For this review, take the finished solid that the model builds, in its own axes (mm). A direction names the side the tool comes from. Coordinates: 2 decimals unless noted, no trailing zeros. Write each loop counter-clockwise with the first axis right and the second up, starting at its lowest first coordinate (ties: lowest second). Pieces come first, ordered by that corner, then holes. Notation, with made-up numbers: M -13,40.5 L 44,40.5 A13 cw 44,47.5 Z; hole C -30.75,22 d10. An arc over 180 degrees is marked long. One line per question, with ' | ' between items.
from build123d import *

# Parameters (mm, degrees)
BOSS_EXTRUDE1_DEPTH  = 20
SKETCH2_W            = 20
SKETCH2_H            = 22
BOSS_EXTRUDE2_DEPTH  = 2.2
BOSS_EXTRUDE3_DEPTH  = 2
SKETCH5_R            = 2.5
BOSS_EXTRUDE4_DEPTH  = 4
FILLET1_R            = 1
FILLET2_R            = 1
FILLET1_OF_MIRROR1_R = 1
FILLET2_OF_MIRROR1_R = 1
SKETCH6_R            = 2
CUT_EXTRUDE1_DEPTH   = 38.406182644


with BuildPart() as part:
    # Sketch1 → Boss-Extrude1 (new, symmetric)
    with BuildSketch(Plane.XY):
        Polygon((-3, 0), (3, 0), (3, -2), (5.3, -2), (5.3, -3.62), (2.8, -6.1), (-2.8, -6.1), (-5.3, -3.62), (-5.3, -2), (-3, -2), align=None)
    extrude(amount=BOSS_EXTRUDE1_DEPTH, both=True)

    # Sketch2 → Boss-Extrude2 (add)
    with BuildSketch(Plane(origin=(0, 0, 0), x_dir=(1, 0, 0), z_dir=(0, 1, 0))):
        Rectangle(SKETCH2_W, SKETCH2_H)
    extrude(amount=BOSS_EXTRUDE2_DEPTH)

    # Sketch4 → Boss-Extrude3 (add)
    with BuildSketch(Plane.XY.offset(11)):
        with BuildLine():
            Line((-3, 0), (3, 0))
            Line((3, 0), (10, 0))
            Line((10, 0), (10, 2.2))
            Line((10, 2.2), (-7.139065943, 24.501455527))
            ThreePointArc((-7.139065943, 24.501455527), (-14.108916266, 25.991854595), (-16.69750329, 19.351122698))
            Line((-16.69750329, 19.351122698), (-10, 0))
            Line((-10, 0), (-3, 0))
        make_face()
    boss_extrude3 = extrude(amount=-BOSS_EXTRUDE3_DEPTH)

    # Sketch5 → Boss-Extrude4 (add)
    with BuildSketch(Plane(origin=(0, 0, 9), x_dir=(-1, 0, 0), z_dir=(0, 0, -1))):
        with Locations(Location((11.5, 21.15, 0), (0, 0, 180))):
            Circle(SKETCH5_R)
    boss_extrude4 = extrude(amount=BOSS_EXTRUDE4_DEPTH)

    # Fillet1
    fillet1_edges = [part.edges().sort_by_distance(p)[0] for p in [
        (-14, 21.15, 5),
    ]]
    fillet(fillet1_edges, radius=FILLET1_R)

    # Fillet2
    fillet2_edges = [part.edges().sort_by_distance(p)[0] for p in [
        (1.430467029, 13.350727763, 11),
        (-14.108916266, 25.991854595, 11),
        (-13.348751645, 9.675561349, 11),
    ]]
    fillet(fillet2_edges, radius=FILLET2_R)

    # Mirror1: Boss-Extrude3, Boss-Extrude4 across plane
    add(boss_extrude3.mirror(Plane.XY))
    add(boss_extrude4.mirror(Plane.XY))

    # Fillet1 of Mirror1
    fillet1_of_mirror1_edges = [part.edges().sort_by_distance(p)[0] for p in [
        (-14, 21.15, -5),
    ]]
    fillet(fillet1_of_mirror1_edges, radius=FILLET1_OF_MIRROR1_R)

    # Fillet2 of Mirror1
    fillet2_of_mirror1_edges = [part.edges().sort_by_distance(p)[0] for p in [
        (1.430467029, 13.350727763, -11),
        (-14.108916266, 25.991854595, -11),
        (-13.348751645, 9.675561349, -11),
    ]]
    fillet(fillet2_of_mirror1_edges, radius=FILLET2_OF_MIRROR1_R)

    # Sketch6 → Cut-Extrude1 (cut, through all)
    with BuildSketch(Plane(origin=(0, 0, 0), x_dir=(1, 0, 0), z_dir=(0, 1, 0))):
        with Locations(Location((0, 16, 0), (0, 0, 270))):
            Circle(SKETCH6_R)
        with Locations(Location((0, -16, 0), (0, 0, 270))):
            Circle(SKETCH6_R)
    extrude(amount=-CUT_EXTRUDE1_DEPTH, mode=Mode.SUBTRACT)


solid = part.part
1) Insertion check: pin 1 Ø5.5 at (x, z) = (3.5, 0.5) entering from +Y; pin 2 Ø10 at (x, y) = (-10, 9.5) entering from -Z; pin 3 Ø8 at (x, y) = (-3.5, 16.5) entering from +Z; pin 4 Ø4 at (x, z) = (4, -7) entering from -Y. Each pin has a flat end and moves straight along its axis. Give the tip position at first contact, or say it passes through.
Responses:
pin 1: y = 2.2 | pin 2: z = -11 | pin 3: z = 11 | pin 4: y = -6.1
2) To check wall thickness, follow line 1 along Z through (x, y) = (-4.5, 9); line 2 along X through (y, z) = (-1.75, 16); line 3 along X through (y, z) = (-3, 16). State the ranges of each line that lie inside material, in increasing order. Write a range as [from, to].
Responses:
line 1: [-11, -9], [9, 11] | line 2: [-3, -2], [2, 3] | line 3: [-5.3, -2], [2, 5.3]
3) Machinability: for faces 1 (the cylindrical face through (-13.998, 21.04, -7.521)), 2 (the flat face through (-6, 10, 11)), 3 (the flat face through (-10, 1, 0)), 4 (the flat face through (-4, -2, 0)), which of the approach directions +Z, -Z, +X, -X, +Y, -Y give a long, thin tool a straight path to every point of the face, cutting with its end or side? Answer none if there is none.
Responses:
face 1: none | face 2: +Z, +X, -X, +Y | face 3: -X, -Y | face 4: +Z, -Z, -X
4) We need section B-B on z = 13.5. State the section outline as (x, y) points.
Responses:
outline: M -5.3,-3.62 L -2.8,-6.1 L 2.8,-6.1 L 5.3,-3.62 L 5.3,-2 L 3,-2 L 3,0 L -3,0 L -3,-2 L -5.3,-2 Z
5) We need section D-D on x = 0. State how many separate pieces and enclosed holes the cut face has, then the cut area to 3 significant figures.
Responses:
separate pieces: 3 | enclosed holes: 0 | area: 295 mm^2
6) We need section A-A on z = -6.5. State the section outline as (x, y) points.
Responses:
outline: C -11.5,21.15 d5; M -10,0 L -3,0 L -3,-2 L -5.3,-2 L -5.3,-3.62 L -2.8,-6.1 L 2.8,-6.1 L 5.3,-3.62 L 5.3,-2 L 3,-2 L 3,0 L 10,0 L 10,2.2 L -10,2.2 Z
7) The part is to be moulded in two halves that separate along X. For faces 5 (the flat face through (1.55, 13.195, 9.507)), 6 (the flat face through (-13.396, 9.811, 9.507)), 7 (the cylindrical face through (-1.774, -3.007, 16.923)), 8 (the cylindrical face through (-1.2, -3, -17.6)), say which applies: +X half, -X half, draft (parallel to the pull), parting line (faces both ways), or undercut.
Responses:
face 5: +X half | face 6: -X half | face 7: undercut | face 8: undercut
8) We need section C-C on z = -16. State the section outline as (x, y) points.
Responses:
outline: M -5.3,-3.62 L -2.8,-6.1 L -2,-6.1 L -2,0 L -3,0 L -3,-2 L -5.3,-2 Z; M 2,-6.1 L 2.8,-6.1 L 5.3,-3.62 L 5.3,-2 L 3,-2 L 3,0 L 2,0 Z
